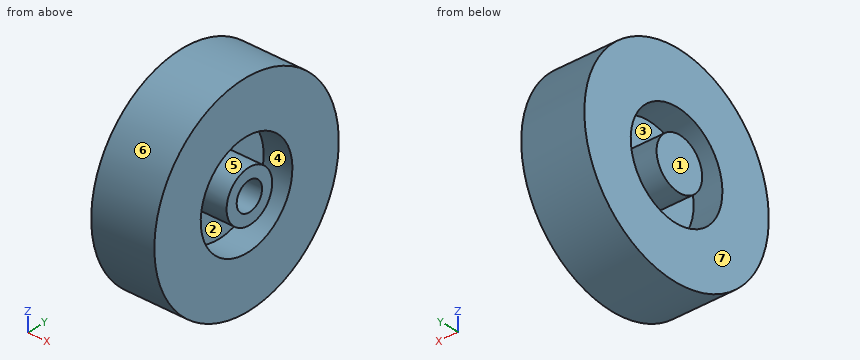
```python
from build123d import *

# Parameters (mm, degrees)
SKETCH2_R          = 5
CUT_EXTRUDE1_DEPTH = 15


with BuildPart() as part:
    # Sketch1 → Revolve1 (revolve)
    with BuildSketch(Plane.XY, mode=Mode.PRIVATE) as revolve1_sk:
        Polygon((-11.2, 18.1), (-1, 18.1), (-1, 9), (-12.2, 9), (-12.2, 0), (12.2, 0), (12.2, 9), (1, 9), (1, 18.1), (11.2, 18.1), (11.2, 36.4), (-11.2, 36.4), align=None)
    revolve(revolve1_sk.sketch.rotate(Axis((0, 0, 0), (1, 0, 0)), 90), axis=Axis((0, 0, 0), (1, 0, 0)))

    # Sketch2 → Cut-Extrude1 (cut)
    with BuildSketch(Plane(origin=(12.2, 0, 0), x_dir=(0, 0, -1), z_dir=(1, 0, 0))):
        Circle(SKETCH2_R)
    extrude(amount=-CUT_EXTRUDE1_DEPTH, mode=Mode.SUBTRACT)


solid = part.part
```
Source: CAD feature listing. Evaluate the final solid. Frame: model axes, mm. Face numbers are marked on the shaded views. A direction names the side the tool comes from. Round coordinates to 2 decimals unless told otherwise and drop trailing zeros. Loops run counter-clockwise (first coordinate to the right, second up) from the corner with the lowest first, then second, coordinate; pieces in that order, holes last. Notation, with made-up numbers: M -28.5,31 L 13.5,31 A29 cw 13.5,53 Z; hole C 49,-17 d5. An arc over 180 degrees is marked long. Use a Markdown table: item, result. Add a question column.
1. Mould query, pull axis Z, two halves, no side actions, for the marked faces 4, 5, 6 and 7. Classes: pulls with the +Z half, pulls with the -Z half, needs draft (parallel to the pull), parting line crosses it, or undercut.
2. Contact query for flat-ended pins moving along their axis: P1, Ø12, axis at x = 1.5, z = 10.5, coming from the +Y side; P2, Ø3, axis at x = 9, y = 6, coming from the -Z side; P3, Ø1, axis at x = -1, z = -2, coming from the +Y side. Output: stop coordinate, or through.
3. Reachability of the marked faces 1, 2 and 3 from +Z, -Z, +X, -X, +Y, -Y: full face, straight path, thin tool, end or side. Return the list, or none.
4. Line query: line 1 (Y direction, x = 5, z = 0); line 2 (Y direction, x = -4.5, z = 0); line 3 (X direction, y = 32, z = -1). Output: solid intervals per line, ascending.
5. Section query C-C on x = -5.25. Return the cut outline in (y, z), then the cut area to 3 significant figures.
6. Section query B-B on z = 0. Return the cut outline in (x, y).
7. Section query A-A on x = 3.5. Return the cut outline in (y, z), then the cut area to 3 significant figures.
Reported:
| question | item | result |
|---|---|---|
| 1 | face 4 | undercut |
| 1 | face 5 | undercut |
| 1 | face 6 | parting line crosses it |
| 1 | face 7 | needs draft |
| 2 | P1 | stops at y = 36.12 |
| 2 | P2 | stops at z = -36.12 |
| 2 | P3 | stops at y = 36.37 |
| 3 | face 1 | +Z, -Z, -X, +Y, -Y |
| 3 | face 2 | +X |
| 3 | face 3 | -X |
| 4 | line 1 | y = -36.4 to -18.1, -9 to -5, 5 to 9, 18.1 to 36.4 |
| 4 | line 2 | y = -36.4 to -18.1, -9 to 9, 18.1 to 36.4 |
| 4 | line 3 | x = -11.2 to 11.2 |
| 5 | outline | C 0,0 d72.8; C 0,0 d18; hole C 0,0 d36.2 |
| 5 | area | 3,390 mm² |
| 6 | outline | M -12.2,-9 L -1,-9 L -1,-18.1 L -11.2,-18.1 L -11.2,-36.4 L 11.2,-36.4 L 11.2,-18.1 L 1,-18.1 L 1,-9 L 12.2,-9 L 12.2,-5 L -2.8,-5 L -2.8,5 L 12.2,5 L 12.2,9 L 1,9 L 1,18.1 L 11.2,18.1 L 11.2,36.4 L -11.2,36.4 L -11.2,18.1 L -1,18.1 L -1,9 L -12.2,9 Z |
| 7 | outline | C 0,0 d72.8; C 0,0 d18; hole C 0,0 d36.2; hole C 0,0 d10 |
| 7 | area | 3,310 mm² |
